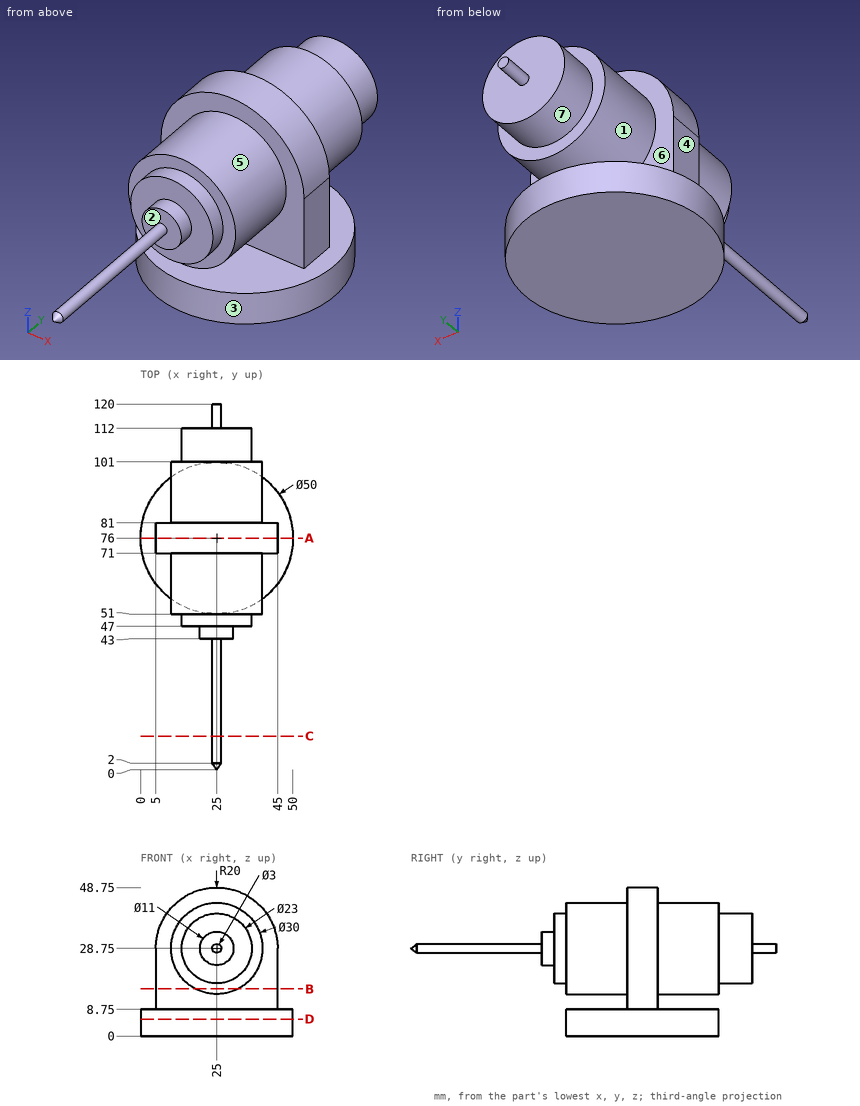
Design review of the part shown in the three views and the two pictorial views. Dimensions are in mm from the part's minimum x, y and z. A direction names the side the tool comes from. Coordinates: 2 decimals unless noted, no trailing zeros. Order: outer loops, then holes, each group sorted by start corner. A loop starts at its lowest first (then second) coordinate and runs counter-clockwise, first axis right, second up. Notation, with made-up numbers: (-23, -28) - (23, -28) arc R11 ccw to (23, -21) - close; hole circle Ø6 at (48.5, -8). An arc over 180 degrees is marked (long way). One line per question, with ' | ' between items.
Q1. To check wall thickness, follow line 1 along Y through (x, z) = (18, 36); line 2 along Z through (x, y) = (46.5, 63.5); line 3 along X through (y, z) = (75.5, 3) (3 decimals). State the ranges of each line that lie inside material, in increasing order.
Answer key:
line 1: y = 47 to 112 | line 2: z = 0 to 8.75 | line 3: x = 0.005 to 49.995
Q2. Consider section D-D, the plane z = 5.5. Give the boundary of the cut face in (x, y), then the cut area to 3 significant figures.
Answer key:
outline: circle Ø50 at (25, 76) | area: 1,960 mm2
Q3. For the marked faces 1, 2 and 3, list the 3-axis set-ups (+Z, -Z, +X, -X, +Y, -Y) from which the entire face can be reached by the end or side of a thin tool; tool diameter is ignored.
Answer key:
face 1: +Y | face 2: -Y | face 3: -Z
Q4. Consider section C-C, the plane y = 11. Give the boundary of the cut face in (x, z).
Answer key:
outline: circle Ø3 at (25, 28.75)
Q5. The part is to be moulded in two halves that separate along Z. For the marked faces 4, 5, 6 and 7, say which applies: +Z half, -Z half, draft (parallel to the pull), parting line (faces both ways), or undercut.
Answer key:
face 4: draft | face 5: undercut | face 6: undercut | face 7: parting line
Q6. Consider section A-A, the plane y = 76. Give the boundary of the cut face in (x, z), then the cut area to 3 significant figures.
Answer key:
outline: (0, 0) - (50, 0) - (50, 8.75) - (45, 8.75) - (45, 28.75) arc R20 ccw to (5, 28.75) - (5, 8.75) - (0, 8.75) - close | area: 1,870 mm2
Q7. Consider section B-B, the plane z = 15.5. Give the boundary of the cut face in (x, y), then the cut area to 3 significant figures.
Answer key:
outline: (5, 71) - (17.97, 71) - (17.97, 51) - (32.03, 51) - (32.03, 71) - (45, 71) - (45, 81) - (32.03, 81) - (32.03, 101) - (17.97, 101) - (17.97, 81) - (5, 81) - close | area: 962 mm2
Q8. Clearance check with flat-ended pins moving along their axes: pin 1 Ø11 at (y, z) = (76.5, 18.5) entering from +X; pin 2 Ø6 at (x, z) = (32, 13) entering from +Y; pin 3 Ø5 at (x, y) = (13.5, 67) entering from +Z. State where each tip first meets the part, or that it passes through.
Answer key:
pin 1: stops at x = 45 | pin 2: stops at y = 101 | pin 3: stops at z = 40.75
